from build123d import *

# Parameters (mm, degrees)
SKETCH1_W           = 12.7
SKETCH1_H           = 8.89
BOSS_EXTRUDE1_DEPTH = 3.175
SKETCH2_R           = 2.38125
BOSS_EXTRUDE2_DEPTH = 6.35
CUT_EXTRUDE1_REACH  = 19.274
SKETCH4_R           = 1.190625
BOSS_EXTRUDE3_DEPTH = 50.8
FILLET1_R           = 12.7


with BuildPart() as part:
    # Sketch1 → Boss-Extrude1 (new body)
    with BuildSketch(Plane.XY):
        with Locations((-6.35, 4.445)):
            Rectangle(SKETCH1_W, SKETCH1_H)
    extrude(amount=BOSS_EXTRUDE1_DEPTH)

    # Sketch2 → Boss-Extrude2 (add)
    with BuildSketch(Plane(origin=(0, 0, 0), x_dir=(0, 0, -1), z_dir=(1, 0, 0))):
        with BuildLine():
            Line((-3.175, 4.445), (-7.62, 8.89))
            Line((-7.62, 8.89), (-7.62, 11.578578051))
            ThreePointArc((-7.62, 11.578578051), (-1.5875, 17.611078051), (4.445, 11.578578051))
            Line((4.445, 11.578578051), (4.445, 8.89))
            Line((4.445, 8.89), (0, 4.445))
            Line((0, 4.445), (0, 8.89))
            Line((0, 8.89), (-3.175, 8.89))
            Line((-3.175, 8.89), (-3.175, 4.445))
        make_face()
        with Locations((-1.5875, 13.208)):
            Circle(SKETCH2_R, mode=Mode.SUBTRACT)
    extrude(amount=-BOSS_EXTRUDE2_DEPTH)

    # Sketch4 → Cut-Extrude1 (cut, up to next)
    with BuildSketch(Plane(origin=(0, 8.89, 0), x_dir=(1, 0, 0), z_dir=(0, 1, 0)), mode=Mode.PRIVATE) as cut_extrude1_sk1:
        with Locations(Location((-7.62, -1.5875, 0), (0, 0, 270))):
            Circle(SKETCH4_R)
    cut_extrude1_tool1 = extrude(cut_extrude1_sk1.sketch, amount=-CUT_EXTRUDE1_REACH, mode=Mode.PRIVATE) & part.part
    add(cut_extrude1_tool1.solids().sort_by_distance((-7.62, 8.89, 1.5875))[0], mode=Mode.SUBTRACT)

    # Sketch5 → Boss-Extrude3 (add)
    with BuildSketch(Plane(origin=(0, 0, 0), x_dir=(0, 0, -1), z_dir=(1, 0, 0))):
        Polygon((-7.416824551, 5.296838174), (-10.387538025, 5.296838174), (-10.387538025, 0), (0, 0), (7.212538025, 0), (7.212538025, 5.296838174), (4.241824551, 5.296838174), (4.241824551, 3.895558234), (0, 3.895558234), (-3.175, 3.895558234), (-7.416824551, 3.895558234), align=None)
    extrude(amount=BOSS_EXTRUDE3_DEPTH)

    # Fillet1
    # the kernel refuses this fillet: 12.7 mm, written as the material it adds along each edge
    with BuildSketch(Plane(origin=(0, 32.528773329, 0), x_dir=(-1, 0, 0), z_dir=(0, -1, 0))) as fillet1_piece_1_section:
        with BuildLine():
            CenterArc((11.453286038, 12.7), FILLET1_R, 205.599864758, 64.400135242)
            Line((0, 7.212538025), (0, 0))
            Line((0, 0), (11.453286038, 0))
        make_face()
    fillet1_piece_1 = extrude(amount=32.528773329, mode=Mode.PRIVATE)
    fillet1_piece_1 = split(fillet1_piece_1, bisect_by=Plane(origin=(-0.789431936, 5.296838174, -5.756080296), z_dir=(0, -1, 0)), keep=Keep.TOP, mode=Mode.PRIVATE)
    fillet1_piece_1 = split(fillet1_piece_1, bisect_by=Plane(origin=(-0.789431936, 4.596198204, -4.241824551), z_dir=(0, 0, -1)), keep=Keep.TOP, mode=Mode.PRIVATE)
    add(fillet1_piece_1)
    with BuildSketch(Plane(origin=(0, 3.895558234, 0), x_dir=(-1, 0, 0), z_dir=(0, -1, 0))) as fillet1_piece_2:
        with BuildLine():
            CenterArc((11.453286038, 12.7), FILLET1_R, 205.599864758, 64.400135242)
            Line((0, 7.212538025), (0, 0))
            Line((0, 0), (11.453286038, 0))
        make_face()
    extrude(amount=3.895558234)


solid = part.part
Work out the finished part from the listing and answer in its coordinate system (mm). A direction names the side the tool comes from. Round coordinates to 2 decimals unless told otherwise and drop trailing zeros. Loops run counter-clockwise (first coordinate to the right, second up) from the corner with the lowest first, then second, coordinate; pieces in that order, holes last. Notation, with made-up numbers: (5, 51) - (60, 51) arc R20 ccw to (60, 76) - close; hole circle Ø6 at (11, -16). An arc over 180 degrees is marked (long way). Use one line per item in the form item = value. Start each with the question number.
(1) Find section A-A on y = 2.75. Determine the outline of the cut face in (x, z) (1 decimal).
(2) Consider line 1 (Y direction, x = 8.5, z = 6.5); line 2 (X direction, y = 12.5, z = 6.5); line 3 (Z direction, x = -9, y = 4.5) (3 decimals). Determine where each line is inside the solid, lowest interval first.
(3) Flat-ended cylindrical pins translate along their axes: P1, Ø1.4, axis at x = -7.62, z = 1.59, coming from the +Y side; P2, Ø2.5, axis at x = -4.5, y = 2.5, coming from the +Z side (3 decimals); P3, Ø1.6, axis at y = 3, z = 5.5, coming from the -X side; P4, Ø2, axis at x = -2, y = 10.5, coming from the +Z side. Find the tip coordinate at first contact, or state that the pin passes through.
(4) Determine the mould class of faces 5 (the face through (26, 3.896, 2)), 6 (the face through (25, 3, 10.388)), 7 (the face through (-12.7, 4, 2)) for opening direction Z: +Z half, -Z half, draft (parallel to the pull), parting line (faces both ways), or undercut.
(5) Find section C-C on y = 12.5. Determine the outline of the cut face in (x, z), and give its area (3 significant figures).
(6) Which of the six approach directions +Z, -Z, +X, -X, +Y, -Y give full straight-line access (tool end or side, diameter ignored) to faces 1 (the face through (50.8, 2, 2)), 2 (the face through (-10, 8.89, 2)), 3 (the face through (-3, 10, -4.445)), 4 (the face through (0, 3, 7))?
(7) Find section D-D on x = 46.5. Determine the outline of the cut face in (y, z).
(8) Find section B-B on x = -7.62. Determine the outline of the cut face in (y, z) (3 decimals), and give its area (3 significant figures).
Answer list:
q1.outline = (-12.7, 0) - (-11.5, 0) arc R12.7 cw to (0, -7.2) - (50.8, -7.2) - (50.8, 10.4) - (0, 10.4) - (0, 3.2) - (-12.7, 3.2) - close; hole circle Ø2.4 at (-7.6, 1.6)
q2.line_1 = 0 to 3.9
q2.line_2 = -6.35 to 0
q2.line_3 = 0 to 3.175
q3.P1 = through
q3.P2 = 3.175
q3.P3 = 0
q3.P4 = 7.62
q4.face_5 = undercut
q4.face_6 = +Z half
q4.face_7 = draft
q5.outline = (-6.35, -4.37) - (0, -4.37) - (0, -0.69) - (-6.35, -0.69) - close; (-6.35, 3.86) - (0, 3.86) - (0, 7.55) - (-6.35, 7.55) - close
q5.area = 46.8 mm^2
q6.face_1 = +Z, -Z, +X, +Y, -Y
q6.face_2 = +Z, -Z, -X, +Y
q6.face_3 = -Z, +X, -X, +Y
q6.face_4 = +Z, -X, -Y
q7.outline = (0, -7.21) - (5.3, -7.21) - (5.3, -4.24) - (3.9, -4.24) - (3.9, 7.42) - (5.3, 7.42) - (5.3, 10.39) - (0, 10.39) - close
q8.outline = (0, -0.592) - (3.896, -0.592) - (3.896, 0) - (8.89, 0) - (8.89, 0.397) - (0, 0.397) - close; (0, 2.778) - (8.89, 2.778) - (8.89, 3.175) - (0, 3.175) - close
q8.area = 9.36 mm^2
